from build123d import *

# Parameters (mm, degrees)
BOSS_EXTRUDE1_DEPTH = 8
CUT_EXTRUDE5_DEPTH  = 4
CHAMFER1_SIZE       = 2


with BuildPart() as part:
    # Sketch1 → Boss-Extrude1 (new body)
    with BuildSketch(Plane(origin=(0, 0, 0), x_dir=(1, 0, 0), z_dir=(0, 1, 0))):
        with BuildLine():
            Line((-20, 20), (20, 20))
            ThreePointArc((20, 20), (40, 0), (20, -20))
            Line((20, -20), (-20, -20))
            ThreePointArc((-20, -20), (-40, 0), (-20, 20))
        make_face()
    extrude(amount=BOSS_EXTRUDE1_DEPTH)

    # Sketch2 → Cut-Extrude5 (cut)
    with BuildSketch(Plane(origin=(0, 8, 0), x_dir=(1, 0, 0), z_dir=(0, 1, 0))):
        with BuildLine():
            Line((-10, -11.180339887), (-10, 11.180339887))
            ThreePointArc((-10, 11.180339887), (-6.505403256, 13.515906498), (-2.5, 14.790199458))
            Line((-2.5, 14.790199458), (-2.5, -14.790199458))
            ThreePointArc((-2.5, -14.790199458), (-6.505403256, -13.515906498), (-10, -11.180339887))
        make_face()
        with BuildLine():
            Line((10, -11.180339887), (10, 11.180339887))
            ThreePointArc((10, 11.180339887), (6.505403256, 13.515906498), (2.5, 14.790199458))
            Line((2.5, 14.790199458), (2.5, -14.790199458))
            ThreePointArc((2.5, -14.790199458), (6.505403256, -13.515906498), (10, -11.180339887))
        make_face()
    extrude(amount=-CUT_EXTRUDE5_DEPTH, mode=Mode.SUBTRACT)

    # Chamfer1
    chamfer1_edges = [part.edges().sort_by_distance(p)[0] for p in [
        (40, 8, 0),
        (0, 8, -20),
        (-40, 8, 0),
        (0, 0, -20),
        (40, 0, 0),
        (0, 0, 20),
        (-40, 0, 0),
        (0, 8, 20),
    ]]
    chamfer(chamfer1_edges, length=CHAMFER1_SIZE)


solid = part.part
Geometry check sheet. Reference: the model listing, model coordinates, mm. A direction names the side the tool comes from. Round coordinates to 2 decimals unless told otherwise and drop trailing zeros. Loops run counter-clockwise (first coordinate to the right, second up) from the corner with the lowest first, then second, coordinate; pieces in that order, holes last.
Item 1: Gauge pin test, flat ends, axial feed: pin 1 (2.5 mm diameter, centred on x = -5, z = -7, fed in from +Y); pin 2 (2 mm diameter, centred on y = 6, z = -6.5, fed in from +X); pin 3 (2 mm diameter, centred on y = 5.5, z = 5.5, fed in from -X); pin 4 (1.5 mm diameter, centred on x = -11, y = 6.5, fed in from -Z). Record the tip position at first contact, or that the pin passes through.
Item 2: Cross-section at B-B on z = 0. Record the boundary of the cut face in (x, y), then the cut area to 3 significant figures.
Item 3: Mould release check, pull along Z, two halves, no side actions. Record for faces 1 (the flat face through (1, 0, 0)), 2 (the cylindrical face through (-40, 4, 0)), 3 (the cylindrical face through (6.56, 6.03, -13.49)), 4 (the flat face through (0, 7, 19)): pulls with the +Z half, pulls with the -Z half, needs draft (parallel to the pull), parting line crosses it, or undercut.
Item 4: Thickness scan on line 1 (X direction, y = 5.5, z = 0); line 2 (X direction, y = 7, z = -12); line 3 (Y direction, x = -8.5, z = -10). Record the ranges inside material, lowest first.
Item 5: Cross-section at A-A on y = 5. Record the boundary of the cut face in (x, z).
Item 6: Access from +Z, -Z, +X, -X, +Y, -Y to the whole of each face (thin tool, end or side, straight path). Record for faces 5 (the cylindrical face through (40, 4, 0)), 6 (the flat face through (2.5, 6, 0)).
Item 7: Cross-section at C-C on x = 6. Record the boundary of the cut face in (y, z), then the cut area to 3 significant figures.
Item 8: Cross-section at D-D on y = 0.75. Record the boundary of the cut face in (x, z), then the cut area to 3 significant figures.
Answer sheet:
1. pin 1: stops at y = 4
1. pin 2: stops at x = 39.23
1. pin 3: stops at x = -39.49
1. pin 4: stops at z = -20
2. outline: (-40, 2) - (-38, 0) - (38, 0) - (40, 2) - (40, 6) - (38, 8) - (10, 8) - (10, 4) - (2.5, 4) - (2.5, 8) - (-2.5, 8) - (-2.5, 4) - (-10, 4) - (-10, 8) - (-38, 8) - (-40, 6) - close
2. area: 572 mm2
3. face 1: needs draft
3. face 2: parting line crosses it
3. face 3: undercut
3. face 4: pulls with the +Z half
4. line 1: x = -40 to -10, -2.5 to 2.5, 10 to 40
4. line 2: x = -34.73 to -9, -2.5 to 2.5, 9 to 34.73
4. line 3: y = 0 to 4
5. outline: (-20, -20) - (20, -20) arc R20 ccw to (20, 20) - (-20, 20) arc R20 ccw to start; hole (-10, -11.18) arc R15 ccw to (-2.5, -14.79) - (-2.5, 14.79) arc R15 ccw to (-10, 11.18) - close; hole (2.5, -14.79) arc R15 ccw to (10, -11.18) - (10, 11.18) arc R15 ccw to (2.5, 14.79) - close
6. face 5: +X, +Y, -Y
6. face 6: +Y
7. outline: (0, -18) - (2, -20) - (6, -20) - (8, -18) - (8, -13.75) - (4, -13.75) - (4, 13.75) - (8, 13.75) - (8, 18) - (6, 20) - (2, 20) - (0, 18) - close
7. area: 202 mm2
8. outline: (-20, -18.75) - (20, -18.75) arc R18.75 ccw to (20, 18.75) - (-20, 18.75) arc R18.75 ccw to start
8. area: 2,600 mm2
